Part model, mm, in its own coordinate system. Face numbers are marked on the shaded views. A direction names the side the tool comes from. Give positions to 0.01 mm unless a question says otherwise; leave off trailing zeros. Order: outer loops, then holes, each group sorted by start corner. A loop starts at its lowest first (then second) coordinate and runs counter-clockwise, first axis right, second up. Notation, with made-up numbers: (37.5, -18) - (71.5, -18) arc R27 ccw to (71.5, 7) - close; hole circle Ø9 at (11, -1.75). An arc over 180 degrees is marked (long way). Use a Markdown table: item, result. Add a question column.
Autodesk Inventor part; units mm, degrees
ref_plane "YZ Plane" through (0, 0, 0) normal (1, 0, 0) x (0, 1, 0)
ref_plane "XZ Plane" through (0, 0, 0) normal (0, 1, 0) x (-1, 0, 0)
ref_plane "XY Plane" through (0, 0, 0) normal (0, 0, 1) x (1, 0, 0)
sketch "Sketch1" plane through (0, 0, 0) normal (0, 0, 1) x (1, 0, 0)
  arc A0 (-59.9, 42.7) -> (-63.8, 38.8) centre (-59.9, 38.8) ccw
  arc A1 (63.8, 38.8) -> (59.9, 42.7) centre (59.9, 38.8) ccw
  arc A2 (59.9, -42.7) -> (63.8, -38.8) centre (59.9, -38.8) ccw
  arc A3 (59.9, -42.8) -> (63.9, -38.8) centre (59.9, -38.8) ccw
  arc A4 (-63.9, -38.8) -> (-59.9, -42.8) centre (-59.9, -38.8) ccw
  line L0 (-63.8, 38.8) -> (-63.9, -38.8)
  line L1 (-59.9, -42.8) -> (59.9, -42.8)
  line L2 (63.9, -38.8) -> (63.8, 38.8)
  line L3 (59.9, 42.7) -> (-59.9, 42.7)
  line L4 (-63.795, 42.7001) -> (63.9, 42.7001)
  line L5 (63.9, 42.7001) -> (63.9, -42.8)
  line L6 (63.9, -42.8) -> (-63.795, -42.8)
  line L7 (-63.795, -42.8) -> (-63.795, 42.7001)
  point P0 (0, 0)
extrude "Extrusion1" add sketch "Sketch1" along normal blind 2 contours L3 A1 L2 A3 L1 A4 L7 A0 | A0 L7 L4 | L4 L5 L2 A1 | A4 L6 L7 | L5 L6 A3
fillet "Fillet1" radius 5 4 edges at (63.9, -42.8, 1) (-63.795, 42.7001, 1) (-63.795, -42.8, 1) (63.9, 42.7001, 1)
sketch "Sketch2" plane through (0, 0, 0) normal (0, 0, -1) x (-1, 0, 0)
  line L0 (-65.9327, 44.5429) -> (66.5944, 44.5429) construction
  line L1 (66.5944, 44.5429) -> (66.5944, -45.2784) construction
  line L2 (66.5944, -45.2784) -> (-65.9327, -45.2784) construction
  line L3 (-65.9327, -45.2784) -> (-65.9327, 44.5429) construction
  arc A0 (-59.9, 42.7) -> (-63.8, 38.8) centre (-59.9, 38.8) ccw
  arc A1 (63.8, 38.8) -> (59.9, 42.7) centre (59.9, 38.8) ccw
  arc A2 (59.9, -42.7) -> (63.8, -38.8) centre (59.9, -38.8) ccw
  arc A3 (-63.8, -38.8) -> (-59.9, -42.7) centre (-59.9, -38.8) ccw
  circle A4 centre (48.3844, 34.4729) radius 5.5
  circle A5 centre (48.3844, 15.1929) radius 5.5
  line L4 (66.5944, 25.2629) -> (66.5944, -64.5584) construction
  circle A6 centre (48.3844, -4.0871) radius 5.5
  line L5 (66.5944, 5.9829) -> (66.5944, -83.8384) construction
  circle A7 centre (48.3844, -23.3671) radius 5.5
  line L6 (66.5944, -13.2971) -> (66.5944, -103.1184) construction
  circle A8 centre (28.4944, 34.4729) radius 5.5
  line L7 (46.7044, 44.5429) -> (46.7044, -45.2784) construction
  circle A9 centre (28.4944, 15.1929) radius 5.5
  line L8 (46.7044, 25.2629) -> (46.7044, -64.5584) construction
  circle A10 centre (28.4944, -4.0871) radius 5.5
  line L9 (46.7044, 5.9829) -> (46.7044, -83.8384) construction
  circle A11 centre (28.4944, -23.3671) radius 5.5
  line L10 (46.7044, -13.2971) -> (46.7044, -103.1184) construction
  circle A12 centre (8.6044, 34.4729) radius 5.5
  line L11 (26.8144, 44.5429) -> (26.8144, -45.2784) construction
  circle A13 centre (8.6044, 15.1929) radius 5.5
  line L12 (26.8144, 25.2629) -> (26.8144, -64.5584) construction
  circle A14 centre (8.6044, -4.0871) radius 5.5
  line L13 (26.8144, 5.9829) -> (26.8144, -83.8384) construction
  circle A15 centre (8.6044, -23.3671) radius 5.5
  line L14 (26.8144, -13.2971) -> (26.8144, -103.1184) construction
  circle A16 centre (-11.2856, 34.4729) radius 5.5
  line L15 (6.9244, 44.5429) -> (6.9244, -45.2784) construction
  circle A17 centre (-11.2856, 15.1929) radius 5.5
  line L16 (6.9244, 25.2629) -> (6.9244, -64.5584) construction
  circle A18 centre (-11.2856, -4.0871) radius 5.5
  line L17 (6.9244, 5.9829) -> (6.9244, -83.8384) construction
  circle A19 centre (-11.2856, -23.3671) radius 5.5
  line L18 (6.9244, -13.2971) -> (6.9244, -103.1184) construction
  circle A20 centre (-31.1756, 34.4729) radius 5.5
  line L19 (-12.9656, 44.5429) -> (-12.9656, -45.2784) construction
  circle A21 centre (-31.1756, 15.1929) radius 5.5
  line L20 (-12.9656, 25.2629) -> (-12.9656, -64.5584) construction
  circle A22 centre (-31.1756, -4.0871) radius 5.5
  line L21 (-12.9656, 5.9829) -> (-12.9656, -83.8384) construction
  circle A23 centre (-31.1756, -23.3671) radius 5.5
  line L22 (-12.9656, -13.2971) -> (-12.9656, -103.1184) construction
  circle A24 centre (-51.0656, 34.4729) radius 5.5
  line L23 (-32.8556, 44.5429) -> (-32.8556, -45.2784) construction
  circle A25 centre (-51.0656, 15.1929) radius 5.5
  line L24 (-32.8556, 25.2629) -> (-32.8556, -64.5584) construction
  circle A26 centre (-51.0656, -4.0871) radius 5.5
  line L25 (-32.8556, 5.9829) -> (-32.8556, -83.8384) construction
  circle A27 centre (-51.0656, -23.3671) radius 5.5
  line L26 (-32.8556, -13.2971) -> (-32.8556, -103.1184) construction
  point P0 (0, 0)
  point P1 (59.9, 19.52)
  point P2 (59.9, 0.24)
  point P3 (59.9, -19.04)
  point P4 (40.01, 38.8)
  point P5 (40.01, 19.52)
  point P6 (40.01, 0.24)
  point P7 (40.01, -19.04)
  point P8 (20.12, 38.8)
  point P9 (20.12, 19.52)
  point P10 (20.12, 0.24)
  point P11 (20.12, -19.04)
  point P12 (0.23, 38.8)
  point P13 (0.23, 19.52)
  point P14 (0.23, 0.24)
  point P15 (0.23, -19.04)
  point P16 (-19.66, 38.8)
  point P17 (-19.66, 19.52)
  point P18 (-19.66, 0.24)
  point P19 (-19.66, -19.04)
  point P20 (-39.55, 38.8)
  point P21 (-39.55, 19.52)
  point P22 (-39.55, 0.24)
  point P23 (-39.55, -19.04)
  dimension "d10" = 11
  dimension "d17" = 19.28
  dimension "d20" = 19.89
  dimension "d24" = 18.21
  dimension "d25" = 10.07
  dimension "d26" = 132.5272
extrude "Extrusion2" cut sketch "Sketch2" against normal blind 2
sketch "Sketch3" plane through (0, 0, 0) normal (0, 0, -1) x (-1, 0, 0)
  circle A0 centre (-51.0656, -4.0871) radius 5.5
  circle A1 centre (-51.0656, 34.4729) radius 5.5
  circle A2 centre (-31.1756, -4.0871) radius 5.5
  circle A3 centre (-31.1756, 34.4729) radius 5.5
  circle A4 centre (-11.2856, -4.0871) radius 5.5
  circle A5 centre (-11.2856, 34.4729) radius 5.5
  circle A6 centre (8.6044, -4.0871) radius 5.5
  circle A7 centre (8.6044, 34.4729) radius 5.5
  circle A8 centre (28.4944, -4.0871) radius 5.5
  circle A9 centre (28.4944, 34.4729) radius 5.5
  circle A10 centre (48.3844, -4.0871) radius 5.5
  circle A11 centre (48.3844, 34.4729) radius 5.5
  circle A12 centre (48.3844, 15.1929) radius 5.5
  circle A13 centre (48.3844, -23.3671) radius 5.5
  circle A14 centre (28.4944, 15.1929) radius 5.5
  circle A15 centre (28.4944, -23.3671) radius 5.5
  circle A16 centre (8.6044, 15.1929) radius 5.5
  circle A17 centre (8.6044, -23.3671) radius 5.5
  circle A18 centre (-11.2856, 15.1929) radius 5.5
  circle A19 centre (-11.2856, -23.3671) radius 5.5
  circle A20 centre (-31.1756, 15.1929) radius 5.5
  circle A21 centre (-31.1756, -23.3671) radius 5.5
  circle A22 centre (-51.0656, 15.1929) radius 5.5
  circle A23 centre (-51.0656, -23.3671) radius 5.5
  arc A24 (-58.9, 42.7001) -> (-63.9, 37.7001) centre (-58.9, 37.7001) ccw
  line L0 (-58.9, 42.7001) -> (58.795, 42.7001)
  arc A25 (63.795, 37.7001) -> (58.795, 42.7001) centre (58.795, 37.7001) ccw
  line L1 (63.795, 37.7001) -> (63.795, -37.8)
  arc A26 (58.795, -42.8) -> (63.795, -37.8) centre (58.795, -37.8) ccw
  line L2 (58.795, -42.8) -> (-58.9, -42.8)
  arc A27 (-63.9, -37.8) -> (-58.9, -42.8) centre (-58.9, -37.8) ccw
  line L3 (-63.9, -37.8) -> (-63.9, 37.7001)
  line L4 (58.795, 40.2001) -> (-58.9, 40.2001)
  arc A28 (-58.9, 40.2001) -> (-61.4, 37.7001) centre (-58.9, 37.7001) ccw
  line L5 (-61.4, 37.7001) -> (-61.4, -37.8)
  arc A29 (-61.4, -37.8) -> (-58.9, -40.3) centre (-58.9, -37.8) ccw
  line L6 (-58.9, -40.3) -> (58.795, -40.3)
  arc A30 (58.795, -40.3) -> (61.295, -37.8) centre (58.795, -37.8) ccw
  line L7 (61.295, -37.8) -> (61.295, 37.7001)
  arc A31 (61.295, 37.7001) -> (58.795, 40.2001) centre (58.795, 37.7001) ccw
  point P0 (0, 0)
  dimension "d27" = 2.5
extrude "Extrusion3" add sketch "Sketch3" along normal blind 30 contours L0 A25 L1 A26 L2 A27 L3 A24
properties part number "00_Rack_Eppendorf_Tubes"
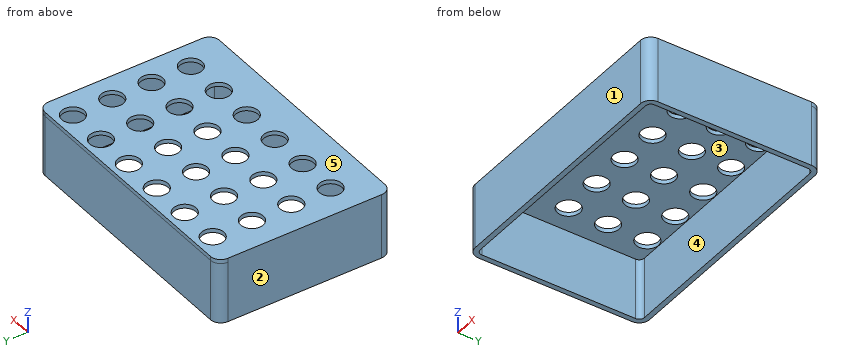
1. Drill centre lines: probe 1 along X at (y, z) = (-18.5, -22.5) (3 decimals); probe 2 along Y at (x, z) = (-23.5, -15.5); probe 3 along Z at (x, y) = (-44, 21). Where is each one in solid material? Low to high. Write a range as [from, to].
2. Cut at C-C (z = -27). Write the cut outline in (x, y) (3 decimals).
3. Cut at B-B (x = -15.5). Write the cut outline in (y, z), plus the area to 3 significant figures.
4. Tool access for the marked faces 4 and 5: list every direction of +Z, -Z, +X, -X, +Y, -Y with a clear straight run to the whole face (end or side of a thin tool).
5. Cut at A-A (y = -7.5). State how many separate pieces and enclosed holes the cut face has, plus the area to 3 significant figures.
6. Pin check, flat tips, straight feed: P1, Ø10, axis at x = 51.07, y = -23.37, coming from the +Z side; P2, Ø17.5, axis at x = 31.18, y = -23.37, coming from the -Z side. Stop position of each tip, or through.
7. Mould opens along Y. For the marked faces 1, 2 and 3 say: released by +Y, released by -Y, zero draft, split by the parting line, or undercut.
8. Cut at D-D (x = 47). Write the cut outline in (y, z), plus the area to 3 significant figures.
Responses:
| question | item | result |
|---|---|---|
| 1 | probe 1 | x = [-63.795, -61.295], [61.4, 63.9] |
| 1 | probe 2 | y = [-42.8, -40.3], [40.2, 42.7] |
| 1 | probe 3 | z = [0, 2] |
| 2 | outline | (-63.795, -37.8) arc R5 ccw to (-58.795, -42.8) - (58.9, -42.8) arc R5 ccw to (63.9, -37.8) - (63.9, 37.7) arc R5 ccw to (58.9, 42.7) - (-58.795, 42.7) arc R5 ccw to (-63.795, 37.7) - close; hole (-61.295, -37.8) arc R2.5 ccw to (-58.795, -40.3) - (58.9, -40.3) arc R2.5 ccw to (61.4, -37.8) - (61.4, 37.7) arc R2.5 ccw to (58.9, 40.2) - (-58.795, 40.2) arc R2.5 ccw to (-61.295, 37.7) - close |
| 3 | outline | (-42.8, -30) - (-40.3, -30) - (-40.3, 0) - (40.2, 0) - (40.2, -30) - (42.7, -30) - (42.7, 2) - (-42.8, 2) - close |
| 3 | area | 321 mm² |
| 4 | face 4 | -Z |
| 4 | face 5 | +Z, +X, -X, +Y, -Y |
| 5 | separate pieces | 7 |
| 5 | enclosed holes | 0 |
| 5 | area | 302 mm² |
| 6 | P1 | passes through |
| 6 | P2 | stops at z = 0 |
| 7 | face 1 | released by -Y |
| 7 | face 2 | zero draft |
| 7 | face 3 | undercut |
| 8 | outline | (-42.8, -30) - (-40.3, -30) - (-40.3, 0) - (-27.07, 0) - (-27.07, 2) - (-42.8, 2) - close; (-19.66, 0) - (-7.79, 0) - (-7.79, 2) - (-19.66, 2) - close; (-0.38, 0) - (11.49, 0) - (11.49, 2) - (-0.38, 2) - close; (18.9, 0) - (30.77, 0) - (30.77, 2) - (18.9, 2) - close; (38.18, 0) - (40.2, 0) - (40.2, -30) - (42.7, -30) - (42.7, 2) - (38.18, 2) - close |
| 8 | area | 262 mm² |
